Geometry check sheet. Reference: the model listing, model coordinates, mm. Give positions to 0.01 mm unless a question says otherwise; leave off trailing zeros. Write each loop counter-clockwise with the first axis right and the second up, starting at its lowest first coordinate (ties: lowest second). Pieces come first, ordered by that corner, then holes. Notation, with made-up numbers: (55, 36.5) -> (99, 36.5) arc R19 cw to (99, 49.5) -> close; hole circle Ø11 at (18.25, 8.5). An arc over 180 degrees is marked (long way). Write item = value, one per line. Start each with the question number.
1. Cross-section at C-C, the plane z = 4. Record the cut outline in (x, y), plus the area to 3 significant figures.
2. Depth check by flat-ended pin: P1, Ø24, axis at x = -6, y = 5, coming from the +Z side; P2, Ø1.5, axis at x = -18, z = 4.5, coming from the +Y side; P3, Ø3, axis at x = 4.5, z = 5.5, coming from the +Y side. Enter the tip coordinate at first touch or a pass-through.
3. Thickness scan on line 1 along Y through (x, z) = (0, 6.75); line 2 along Z through (x, y) = (-1, 10); line 3 along Y through (x, z) = (-12.5, 6.75). Record the ranges inside material, lowest first.
4. Mould release check, pull along X, two halves, no side actions. Record for faces 1 (the flat face through (0, 0, 0)), 2 (the cylindrical face through (-23.977, 1.055, 6.056)), 3 (the cylindrical face through (23.846, 7.509, 4.944)): pulls with the +X half, pulls with the -X half, needs draft (parallel to the pull), parting line crosses it, or undercut.
```python
from build123d import *

# Parameters (mm, degrees)
F0_R     = 25
F1_DEPTH = 10
F2_R     = 24
F3_DEPTH = 8
F4_R     = 0.99999
F5_R     = 1


# Not quite as in the source:
# - a fillet or chamfer is up to 0.001 mm smaller than in the source, because OpenCascade refuses the exact size


with BuildPart() as f1:
    # F0 (on Top) → F1 (new body)
    with BuildSketch(Plane.XY):
        Circle(F0_R)
    extrude(amount=F1_DEPTH)

    # F2 (on face) → F3 (cut)
    with BuildSketch(Plane.XY.offset(10)):
        Circle(F2_R)
    extrude(amount=-F3_DEPTH, mode=Mode.SUBTRACT)

    # F4 (radius 1 in the source; OpenCascade refuses exactly that, so slightly less here)
    f4_edges = [f1.edges().sort_by_distance(p)[0] for p in [
        (-25, 0, 10),
    ]]
    fillet(f4_edges, radius=F4_R)

    # F5
    f5_edges = [f1.edges().sort_by_distance(p)[0] for p in [
        (-25, 0, 0),
    ]]
    fillet(f5_edges, radius=F5_R)


solid = f1.part
```
Answers:
q1.outline = circle Ø50 at (0, 0); hole circle Ø48 at (0, 0)
q1.area = 154 mm^2
q2.P1 = 2
q2.P2 = 18.1
q2.P3 = 24.82
q3.line_1 = -25 to -24, 24 to 25
q3.line_2 = 0 to 2
q3.line_3 = -21.65 to -20.49, 20.49 to 21.65
q4.face_1 = needs draft
q4.face_2 = undercut
q4.face_3 = parting line crosses it
